Job drawing, mm, ordinate dimensions from the low corner. One solid piece. Round coordinates to 2 decimals unless told otherwise and drop trailing zeros. Loops run counter-clockwise (first coordinate to the right, second up) from the corner with the lowest first, then second, coordinate; pieces in that order, holes last.
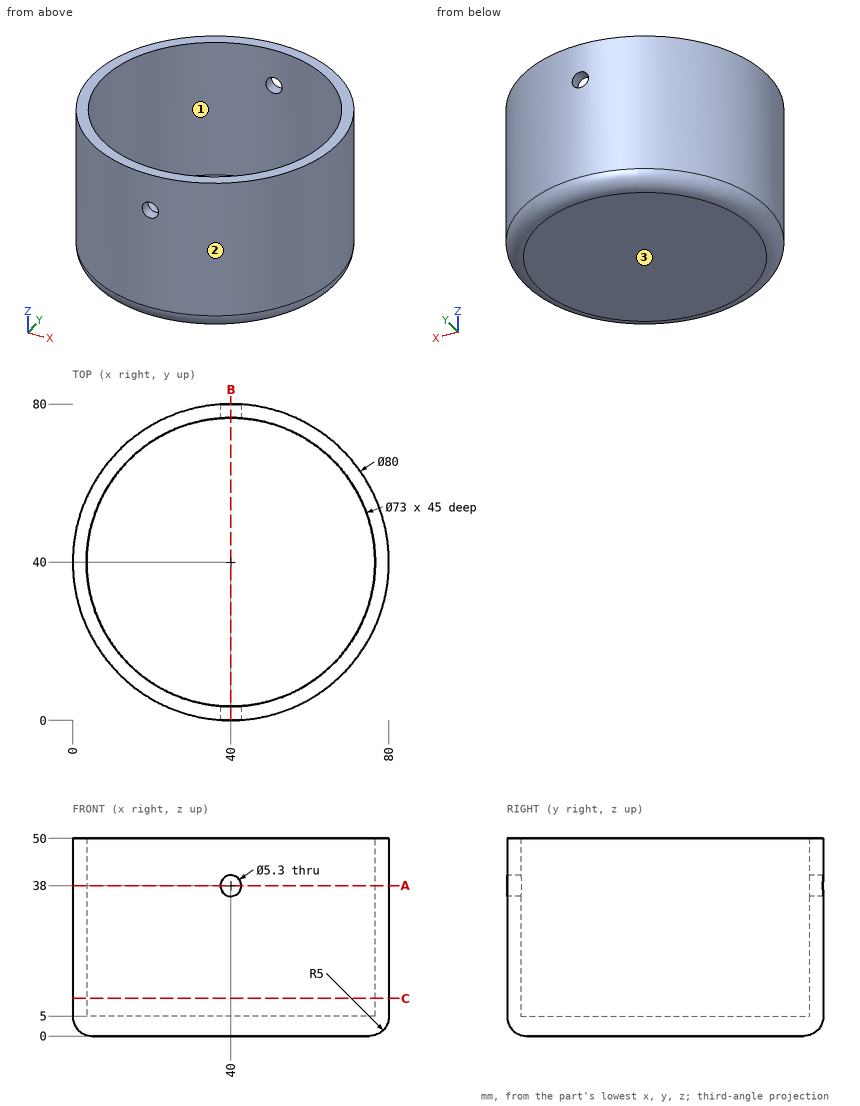
(1) Probe line 1 (Y direction, x = 40, z = 28.5); line 2 (Z direction, x = 44, y = 23.5); line 3 (Y direction, x = 10, z = 14.5). List the from-to ranges inside material, lowest first.
Responses:
line 1: y = 0 to 3.5, 76.5 to 80
line 2: z = 0 to 5
line 3: y = 13.54 to 19.21, 60.79 to 66.46
(2) Slice it at C-C on z = 9.5. List the corners of the cut face in (x, y), plus the area to 3 significant figures.
Responses:
outline: circle Ø80 at (40, 40); hole circle Ø73 at (40, 40)
area: 841 mm2
(3) Pin check, flat tips, straight feed: P1, Ø6, axis at y = 20.5, z = 24.5, coming from the -X side; P2, Ø5, axis at x = 40, z = 38, coming from the -Y side; P3, Ø5, axis at x = 45, z = 14.5, coming from the +Y side; P4, Ø10, axis at x = 58.5, z = 16.5, coming from the -Y side. Stop position of each tip, or through.
Responses:
P1: stops at x = 3.56
P2: passes through
P3: stops at y = 79.92
P4: stops at y = 2.35
(4) Slice it at A-A on z = 38. List the corners of the cut face in (x, y).
Responses:
outline: (37.35, 0.09) - (37.35, 3.6) arc R36.5 cw to (37.35, 76.4) - (37.35, 79.91) arc R40 ccw to start; (42.65, 0.09) arc R40 ccw to (42.65, 79.91) - (42.65, 76.4) arc R36.5 cw to (42.65, 3.6) - close
(5) Pull direction X, two halves, no side cores. Call the marked faces 1, 2 and 3: +X half, -X half, draft (parallel to the pull), parting line (faces both ways), or undercut.
Responses:
face 1: undercut
face 2: parting line
face 3: draft
(6) Slice it at B-B on x = 40. Count the separate pieces of the cut face and the enclosed holes in it, plus the area to 3 significant figures.
Responses:
separate pieces: 3
enclosed holes: 0
area: 667 mm2
